```python
from build123d import *

# Parameters (mm, degrees)
F0_R     = 38.45
F0_R_2   = 35.25
F1_DEPTH = 5
F2_R     = 38.45
F3_DEPTH = 3.2
F5_DEPTH = 25
F6_R     = 5
F7_R     = 1


with BuildPart() as f1:
    # F0 (on Front) → F1 (new body)
    with BuildSketch(Plane.XZ):
        Circle(F0_R)
        Circle(F0_R_2, mode=Mode.SUBTRACT)
    extrude(amount=F1_DEPTH)

    # F2 (on face) → F3 (join)
    with BuildSketch(Plane.XZ.offset(5)):
        Circle(F2_R)
    extrude(amount=F3_DEPTH)

    # F4 (on face) → F5 (cut)
    with BuildSketch(Plane.XZ.offset(8.2)):
        with BuildLine():
            Line((6.4361406616, 1), (1.4361406616, 1))
            ThreePointArc((1.4361406616, 1), (-1.75, 0), (1.4361406616, -1))
            Line((1.4361406616, -1), (6.4361406616, -1))
            ThreePointArc((6.4361406616, -1), (21.2635468628, -16.8975326234), (41.4361406616, -25))
            Line((41.4361406616, -25), (41.4361406616, 25))
            ThreePointArc((41.4361406616, 25), (21.2635468628, 16.8975326234), (6.4361406616, 1))
        make_face()
    extrude(amount=-F5_DEPTH, mode=Mode.SUBTRACT)

    # F6
    f6_edges = [f1.edges().sort_by_distance(p)[0] for p in [
        (31.364819, -4.1, 22.240743),
        (31.364819, -4.1, -22.240743),
        (6.436141, -6.6, -1),
        (6.436141, -6.6, 1),
    ]]
    fillet(f6_edges, radius=F6_R)

    # F7
    f7_edges = [f1.edges().sort_by_distance(p)[0] for p in [
        (1.436141, -6.6, 1),
        (1.436141, -6.6, -1),
        (27.756441, -2.5, 21.72884),
        (27.756441, -2.5, -21.72884),
    ]]
    fillet(f7_edges, radius=F7_R)


solid = f1.part
```
Model file for the job. Use its own axes, mm. A direction names the side the tool comes from. Give positions to 0.01 mm unless a question says otherwise; leave off trailing zeros. Write each loop counter-clockwise with the first axis right and the second up, starting at its lowest first coordinate (ties: lowest second). Pieces come first, ordered by that corner, then holes. Notation, with made-up numbers: M -29,-36 L -3,-36 A29 ccw -3,-15 Z; hole C 81.5,4 d9. An arc over 180 degrees is marked long. Use a Markdown table: item, result.
1) Pin check, flat tips, straight feed: pin 1 (4 mm diameter, centred on y = -4, z = 13, fed in from +X); pin 2 (3 mm diameter, centred on x = -10, y = -4, fed in from +Z); pin 3 (3 mm diameter, centred on x = -12.5, y = -6.5, fed in from -Z). Stop position of each tip, or through.
Responses:
| item | result |
|---|---|
| pin 1 | stops at x = 18.34 |
| pin 2 | stops at z = 37.5 |
| pin 3 | stops at z = -36.84 |
2) Cut at C-C (x = -32.5). List the corners of the cut face in (y, z).
Responses:
| item | result |
|---|---|
| outline | M -8.2,-20.55 L 0,-20.55 L 0,-13.65 L -5,-13.65 L -5,13.65 L 0,13.65 L 0,20.55 L -8.2,20.55 Z |
3) Drill centre lines: line 1 (Z direction, x = 0, y = -6.55); line 2 (Z direction, x = 0, y = -1.9); line 3 (X direction, y = -3.5, z = -30.5). Where is each one in solid material? Low to high. Write a range as from..to.
Responses:
| item | result |
|---|---|
| line 1 | z = -38.45..-1.75, 1.75..38.45 |
| line 2 | z = -38.45..-35.25, 35.25..38.45 |
| line 3 | x = -23.41..-17.67, 17.67..23.41 |
4) Pull direction Z, two halves, no side cores. Call faces 4 (the cylindrical face through (6.06, -6.58, -1.61)), 5 (the flat face through (-35, 0, -6)), 6 (the cylindrical face through (-38.43, -4.04, 1.26)): +Z half, -Z half, draft (parallel to the pull), parting line (faces both ways), or undercut.
Responses:
| item | result |
|---|---|
| face 4 | undercut |
| face 5 | draft |
| face 6 | parting line |
5) Cut at D-D (x = 13). List the corners of the cut face in (y, z).
Responses:
| item | result |
|---|---|
| outline | M -8.2,-36.19 L 0,-36.19 L 0,-32.77 L -5,-32.77 L -5,-9.79 L -8.2,-9.79 Z; M -8.2,9.79 L -5,9.79 L -5,32.77 L 0,32.77 L 0,36.19 L -8.2,36.19 Z |
6) Cut at B-B (z = 0). List the corners of the cut face in (x, y), and give its area (3 significant figures).
Responses:
| item | result |
|---|---|
| outline | M -38.45,-8.2 L -1.75,-8.2 L -1.75,-5 L -35.25,-5 L -35.25,0 L -38.45,0 Z |
| area | 133 mm2 |
7) Cut at A-A (x = 0). List the corners of the cut face in (y, z).
Responses:
| item | result |
|---|---|
| outline | M -8.2,-38.45 L 0,-38.45 L 0,-35.25 L -5,-35.25 L -5,-1.75 L -8.2,-1.75 Z; M -8.2,1.75 L -5,1.75 L -5,35.25 L 0,35.25 L 0,38.45 L -8.2,38.45 Z |
8) Tool access for faces 1 (the cylindrical face through (6.06, -6.58, 1.61)), 2 (the cylindrical face through (-1.75, -6.62, 0.06)), 3 (the flat face through (-4, -5, 0)): list every direction of +Z, -Z, +X, -X, +Y, -Y with a clear straight run to the whole face (end or side of a thin tool).
Responses:
| item | result |
|---|---|
| face 1 | +X, +Y, -Y |
| face 2 | +Y, -Y |
| face 3 | +Y |
